Check sheet for the modelled part. Datum: model origin and axes. Units: mm. A direction names the side the tool comes from. Round coordinates to 2 decimals unless told otherwise and drop trailing zeros. Write each loop counter-clockwise with the first axis right and the second up, starting at its lowest first coordinate (ties: lowest second). Pieces come first, ordered by that corner, then holes. Notation, with made-up numbers: (24, 70.25) -> (64, 70.25) arc R33 cw to (64, 106.25) -> close; hole circle Ø8 at (3, -35). An arc over 180 degrees is marked (long way). Write item = value, one per line.
from build123d import *

# Parameters (mm, degrees)
SKETCH_1_W          = 52
SKETCH_1_H          = 35
SKETCH_1_W_2        = 60
SKETCH_1_H_2        = 28
SKETCH_1_R          = 1.75
SKETCH_1_W_3        = 40
SKETCH_1_H_3        = 20
EXTRUDE_1_DEPTH     = 4
SKETCH_1_3_W        = 4
SKETCH_1_3_H        = 35
EXTRUDE_2_DEPTH     = 34
SKETCH_2_R          = 2.5
CUT_EXTRUDE_1_DEPTH = 85.599054368


with BuildPart() as part:
    # Sketch 1 → Extrude 1 (new body)
    # profile 1 of 2: a face of its own
    with BuildSketch(Plane(origin=(0, 0, 0), x_dir=(1, 0, 0), z_dir=(0, 1, 0))):
        with Locations((0, -31.5)):
            Rectangle(SKETCH_1_W, SKETCH_1_H)
    # profile 2 of 2: a face of its own
    with BuildSketch(Plane(origin=(0, 0, 0), x_dir=(1, 0, 0), z_dir=(0, 1, 0))):
        Rectangle(SKETCH_1_W_2, SKETCH_1_H_2)
        with Locations(Location((-24, -6.007090491, 0), (0, 0, 270))):
            Circle(SKETCH_1_R, mode=Mode.SUBTRACT)
        with Locations(Location((-24, 6.007090491, 0), (0, 0, 270))):
            Circle(SKETCH_1_R, mode=Mode.SUBTRACT)
        with Locations(Location((24, -6.007090491, 0), (0, 0, 270))):
            Circle(SKETCH_1_R, mode=Mode.SUBTRACT)
        with Locations(Location((24, 6.007090491, 0), (0, 0, 270))):
            Circle(SKETCH_1_R, mode=Mode.SUBTRACT)
        Rectangle(SKETCH_1_W_3, SKETCH_1_H_3, mode=Mode.SUBTRACT)
    extrude(amount=EXTRUDE_1_DEPTH)

    # Sketch 1_3 → Extrude 2 (add)
    with BuildSketch(Plane(origin=(0, 0, 0), x_dir=(1, 0, 0), z_dir=(0, 1, 0))):
        with Locations((28, -31.5)):
            Rectangle(SKETCH_1_3_W, SKETCH_1_3_H)
        with Locations((-28, -31.5)):
            Rectangle(SKETCH_1_3_W, SKETCH_1_3_H)
    extrude(amount=EXTRUDE_2_DEPTH)

    # Sketch 2 → Cut-Extrude 1 (cut, through all)
    with BuildSketch(Plane(origin=(30, 0, 0), x_dir=(0, 0, -1), z_dir=(1, 0, 0))):
        with Locations((-41.5, 26.5)):
            Circle(SKETCH_2_R)
        with Locations((-21.5, 26.5)):
            Circle(SKETCH_2_R)
        with Locations((-21.5, 7.5)):
            Circle(SKETCH_2_R)
        with Locations((-41.5, 7.5)):
            Circle(SKETCH_2_R)
    extrude(amount=-CUT_EXTRUDE_1_DEPTH, mode=Mode.SUBTRACT)


solid = part.part
(1) Access from +Z, -Z, +X, -X, +Y, -Y to the whole of each face (thin tool, end or side, straight path). Record for faces 1 (the flat face through (-26, 19, 32)), 2 (the cylindrical face through (-28, 6, 23.5)), 3 (the flat face through (0, 2, -10)).
Worked answers:
face_1 = +Z, -Z, +Y
face_2 = +X, -X
face_3 = +Y, -Y
(2) Go/stop test with flat-tipped pins: P1, Ø10, axis at x = -18, z = 9.5, coming from the +Y side; P2, Ø8, axis at y = 7.5, z = 41.5, coming from the +X side; P3, Ø2, axis at x = 28, y = 17, coming from the -Z side. Record where each tip stops, or that it passes through.
Worked answers:
P1 = 4
P2 = 30
P3 = 14
(3) Sectioned sample at B-B on y = 19. Enter the section's corners in (x, z), then the cut area to 3 significant figures.
Worked answers:
outline = (-30, 14) -> (-26, 14) -> (-26, 49) -> (-30, 49) -> close; (26, 14) -> (30, 14) -> (30, 49) -> (26, 49) -> close
area = 280 mm²
(4) Sectioned sample at C-C on x = -24. Enter the section's corners in (y, z).
Worked answers:
outline = (0, -14) -> (4, -14) -> (4, -7.76) -> (0, -7.76) -> close; (0, -4.26) -> (4, -4.26) -> (4, 4.26) -> (0, 4.26) -> close; (0, 7.76) -> (4, 7.76) -> (4, 49) -> (0, 49) -> close
(5) Sectioned sample at D-D on z = 41.5. Enter the section's corners in (x, y).
Worked answers:
outline = (-30, 0) -> (30, 0) -> (30, 5) -> (26, 5) -> (26, 4) -> (-26, 4) -> (-26, 5) -> (-30, 5) -> close; (-30, 10) -> (-26, 10) -> (-26, 24) -> (-30, 24) -> close; (-30, 29) -> (-26, 29) -> (-26, 34) -> (-30, 34) -> close; (26, 10) -> (30, 10) -> (30, 24) -> (26, 24) -> close; (26, 29) -> (30, 29) -> (30, 34) -> (26, 34) -> close
(6) Release check for a two-part mould opening along X. For faces 4 (the cylindrical face through (28.03, 28.19, 23.34)), 5 (the flat face through (-20, 2, 0)), 6 (the flat face through (-30, 17, 32)) record: pulls with the +X half, pulls with the -X half, needs draft (parallel to the pull), parting line crosses it, or undercut.
Worked answers:
face_4 = needs draft
face_5 = undercut
face_6 = pulls with the -X half
(7) Sectioned sample at A-A on x = -3. Enter the section's corners in (y, z).
Worked answers:
outline = (0, -14) -> (4, -14) -> (4, -10) -> (0, -10) -> close; (0, 10) -> (4, 10) -> (4, 49) -> (0, 49) -> close
(8) Material ranges on L1, parallel to X at y = 15, z = 28; L2, parallel to Z at x = 28, y = 7; L3, parallel to Y at x = 9.5, z = 38, recorded low to high. Write a range as [from, to].
Worked answers:
L1 = [-30, -26], [26, 30]
L2 = [14, 19.05], [23.95, 39.05], [43.95, 49]
L3 = [0, 4]
